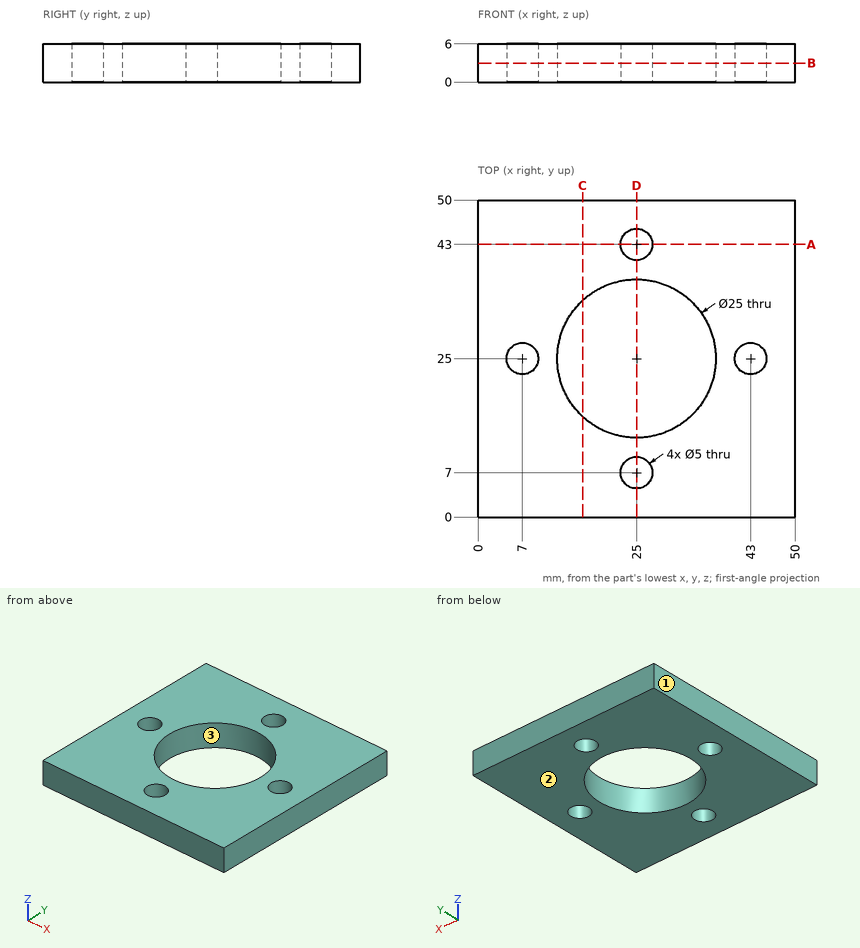
Could you check a few things on this drawing? It's one solid part, dimensions in mm from its lowest x, y, z. Give positions to 0.01 mm unless a question says otherwise; leave off trailing zeros. Loops run counter-clockwise (first coordinate to the right, second up) from the corner with the lowest first, then second, coordinate; pieces in that order, holes last. Notation, with made-up numbers: M -1.5,59.5 L 21.5,59.5 A24 ccw 21.5,89.5 Z; hole C 51.25,-17 d4. An arc over 180 degrees is marked long. Return JSON: item names as keys, results as strings.
Item 1: Please list where these lines run through material, in increasing order: line 1 (Y direction, x = 25, z = 1.4); line 2 (X direction, y = 27, z = 4.1); line 3 (Y direction, x = 29.5, z = 1).
A:
{"line 1": "y = 0 to 4.5, 9.5 to 12.5, 37.5 to 40.5, 45.5 to 50", "line 2": "x = 0 to 5.5, 8.5 to 12.66, 37.34 to 41.5, 44.5 to 50", "line 3": "y = 0 to 13.34, 36.66 to 50"}
Item 2: Imagine slicing it at D-D on x = 25. List the corners of the cut face in (y, z) for me, then the cut area to 3 significant figures.
A:
{"outline": "M 0,0 L 4.5,0 L 4.5,6 L 0,6 Z; M 9.5,0 L 12.5,0 L 12.5,6 L 9.5,6 Z; M 37.5,0 L 40.5,0 L 40.5,6 L 37.5,6 Z; M 45.5,0 L 50,0 L 50,6 L 45.5,6 Z", "area": "90.0 mm^2"}
Item 3: Imagine slicing it at A-A on y = 43. List the corners of the cut face in (x, z) for me, then the cut area to 3 significant figures.
A:
{"outline": "M 0,0 L 22.5,0 L 22.5,6 L 0,6 Z; M 27.5,0 L 50,0 L 50,6 L 27.5,6 Z", "area": "270 mm^2"}
Item 4: Imagine slicing it at B-B on z = 3. List the corners of the cut face in (x, y) for me, then the cut area to 3 significant figures.
A:
{"outline": "M 0,0 L 50,0 L 50,50 L 0,50 Z; hole C 7,25 d5; hole C 25,25 d25; hole C 25,7 d5; hole C 25,43 d5; hole C 43,25 d5", "area": "1,930 mm^2"}
Item 5: I'm going to push a flat-ended pin straight in: pin 1 Ø4 at (x, y) = (7, 25) entering from -Z. Where does the tip first touch, or does it pass through?
A:
{"pin 1": "passes through"}
Item 6: Thinking about a two-plate mould opening in X: for the marked faces 1, 2 and 3, which applies, released by +X, released by -X, zero draft, split by the parting line, or undercut?
A:
{"face 1": "released by -X", "face 2": "zero draft", "face 3": "undercut"}
Item 7: Imagine slicing it at C-C on x = 16.5. List the corners of the cut face in (y, z) for me, then the cut area to 3 significant figures.
A:
{"outline": "M 0,0 L 15.83,0 L 15.83,6 L 0,6 Z; M 34.17,0 L 50,0 L 50,6 L 34.17,6 Z", "area": "190 mm^2"}
